The model under review builds one solid part; all positions refer to its coordinate system, in mm. A direction names the side the tool comes from. Give positions to 0.01 mm unless a question says otherwise; leave off trailing zeros. Loops run counter-clockwise (first coordinate to the right, second up) from the corner with the lowest first, then second, coordinate; pieces in that order, holes last. Notation, with made-up numbers: M 19,-29 L 61,-29 A28 cw 61,-11 Z; hole C 79,-30.5 d3. An arc over 180 degrees is marked long. Return JSON: item names as keys, results as strings.
```python
from build123d import *

# Parameters (mm, degrees)
SKETCH1_W           = 64
SKETCH1_H           = 51
BOSS_EXTRUDE1_DEPTH = 27
SKETCH2_R           = 19
BOSS_EXTRUDE2_DEPTH = 50
SKETCH3_R           = 2.1
BOSS_EXTRUDE3_DEPTH = 6.5
SKETCH4_W           = 12
SKETCH4_H           = 11
BOSS_EXTRUDE4_DEPTH = 50


with BuildPart() as part:
    # Sketch1 → Boss-Extrude1 (new body)
    with BuildSketch(Plane(origin=(0, 0, 0), x_dir=(1, 0, 0), z_dir=(0, 1, 0))):
        with Locations((32, 25.5)):
            Rectangle(SKETCH1_W, SKETCH1_H)
    extrude(amount=BOSS_EXTRUDE1_DEPTH)

    # Sketch2 → Boss-Extrude2 (add)
    with BuildSketch(Plane(origin=(0, 27, 0), x_dir=(1, 0, 0), z_dir=(0, 1, 0))):
        with Locations(Location((32, 25.5, 0), (0, 0, 90))):
            Circle(SKETCH2_R)
    extrude(amount=BOSS_EXTRUDE2_DEPTH)

    # Sketch3 → Boss-Extrude3 (add)
    with BuildSketch(Plane.XZ):
        with Locations(Location((3.5, -3.25, 0), (0, 0, 90))):
            Circle(SKETCH3_R)
        with Locations(Location((60.5, -3.25, 0), (0, 0, 90))):
            Circle(SKETCH3_R)
        with Locations(Location((3.5, -47.75, 0), (0, 0, 90))):
            Circle(SKETCH3_R)
        with Locations(Location((60.5, -47.75, 0), (0, 0, 90))):
            Circle(SKETCH3_R)
    extrude(amount=BOSS_EXTRUDE3_DEPTH)

    # Sketch4 → Boss-Extrude4 (add)
    with BuildSketch(Plane(origin=(64, 0, 0), x_dir=(0, 0, -1), z_dir=(1, 0, 0))):
        with Locations((36, 6.5)):
            Rectangle(SKETCH4_W, SKETCH4_H)
    extrude(amount=BOSS_EXTRUDE4_DEPTH)


solid = part.part
```
1) Consider section B-B on z = -25.5. Write out the cut boundary in (x, y).
From the geometry:
{"outline": "M 0,0 L 64,0 L 64,27 L 51,27 L 51,77 L 13,77 L 13,27 L 0,27 Z"}
2) Consider section C-C on z = -3.25. Write out the cut boundary in (x, y).
From the geometry:
{"outline": "M 0,0 L 1.4,0 L 1.4,-6.5 L 5.6,-6.5 L 5.6,0 L 58.4,0 L 58.4,-6.5 L 62.6,-6.5 L 62.6,0 L 64,0 L 64,27 L 0,27 Z"}
3) Consider section D-D on y = 65.5. Write out the cut boundary in (x, z).
From the geometry:
{"outline": "C 32,-25.5 d38"}
4) Insertion check: pin 1 (8 mm diameter, centred on x = 102, z = -39, fed in from -Y); pin 2 (6 mm diameter, centred on x = 63, y = 24, fed in from +Z); pin 3 (2 mm diameter, centred on y = 43, z = -29.5, fed in from +X); pin 4 (3 mm diameter, centred on x = 83.5, y = 4.5, fed in from -Z). Each pin has a flat end and moves straight along its axis. Give the tip position at first contact, or say it passes through.
From the geometry:
{"pin 1": "y = 1", "pin 2": "z = 0", "pin 3": "x = 50.76", "pin 4": "z = -42"}
5) Wall thickness on L1, parallel to X at y = 17, z = -13.5; L2, parallel to Z at x = 78, y = 2; L3, parallel to Y at x = 6, z = -42.5: over which ranges is each line inside the solid? List them lowest first. Write a range as from..to.
From the geometry:
{"L1": "0..64", "L2": "-42..-30", "L3": "0..27"}
6) The part is to be moulded in two halves that separate along X. For faces 1 (the face through (5.363, -3.204, -2.281)), 2 (the face through (32, 13, 0)), 3 (the face through (50.548, 51.65, -21.381)), 4 (the face through (0, 13, -25)), say which applies: released by +X, released by -X, zero draft, split by the parting line, or undercut.
From the geometry:
{"face 1": "undercut", "face 2": "zero draft", "face 3": "split by the parting line", "face 4": "released by -X"}
7) Consider section A-A on x = 32. Write out the cut boundary in (y, z).
From the geometry:
{"outline": "M 0,-51 L 27,-51 L 27,-44.5 L 77,-44.5 L 77,-6.5 L 27,-6.5 L 27,0 L 0,0 Z"}
8) Tool access review of faces 5 (the face through (53, 27, -26)), 6 (the face through (4.3, -3.2, -45.81)), 7 (the face through (89, 12, -36)), 8 (the face through (89, 6, -42)): name each direction out of +Z, -Z, +X, -X, +Y, -Y from which nothing blocks a thin tool from reaching the whole face with its end or side.
From the geometry:
{"face 5": "+Y", "face 6": "-Y", "face 7": "+Z, -Z, +X, +Y", "face 8": "-Z, +X, +Y, -Y"}
